```python
from build123d import *

# Parameters (mm, degrees)
FILLET1_R               = 1
FILLET2_R               = 1
BOSS_EXTRUDE1_DEPTH     = 7
CUT_EXTRUDE1_REACH      = 12.127
CUT_EXTRUDE1_END_RADIUS = 5.175
SKETCH2_R               = 1.51
SKETCH2_R_2             = 0.51
SKETCH4_R               = 0.75
CUT_EXTRUDE2_DEPTH      = 1.5


with BuildPart() as part:
    # Sketch1 → Revolve1 (revolve)
    with BuildSketch(Plane.XY, mode=Mode.PRIVATE) as revolve1_sk:
        Polygon((0, 0), (3.175, 0), (3.175, -7), (5.175, -7), (5.175, -4.640909091), (5.175, 1.5), (3.5, 1.5), (3.5, 4.5), (1.5, 4.5), (1.5, 1.5), (0, 1.5), align=None)
    revolve(revolve1_sk.sketch.rotate(Axis((0, 1.5, 0), (0, -1, 0)), 180), axis=Axis((0, 1.5, 0), (0, -1, 0)))

    # Fillet1
    fillet1_edges = [part.edges().sort_by_distance(p)[0] for p in [
        (3.5, 1.5, 0),
    ]]
    fillet(fillet1_edges, radius=FILLET1_R)

    # Fillet2
    fillet2_edges = [part.edges().sort_by_distance(p)[0] for p in [
        (5.175, 1.5, 0),
    ]]
    fillet(fillet2_edges, radius=FILLET2_R)

    # Sketch3 → Boss-Extrude1 (add)
    with BuildSketch(Plane.XZ.offset(7)):
        with BuildLine():
            Line((2.313006701, -2.175), (-2.313006701, -2.175))
            ThreePointArc((-2.313006701, -2.175), (0, -3.175), (2.313006701, -2.175))
        make_face()
    extrude(amount=-BOSS_EXTRUDE1_DEPTH)

    # Cut-Extrude1: up to this cylinder (the profile starts inside it)
    cut_extrude1_end = Plane(origin=(0, 0.120549, 0), z_dir=(0, 1, 0)) * Cylinder(CUT_EXTRUDE1_END_RADIUS, 42.18296, mode=Mode.PRIVATE)
    # Sketch2 → Cut-Extrude1 (cut, up to the surface)
    with BuildSketch(Plane.XY, mode=Mode.PRIVATE) as cut_extrude1_sk1:
        with Locations((0, -3.168930556)):
            Circle(SKETCH2_R)
    cut_extrude1_tool1 = extrude(cut_extrude1_sk1.sketch, amount=-CUT_EXTRUDE1_REACH, mode=Mode.PRIVATE) & cut_extrude1_end
    add(cut_extrude1_tool1.solids().sort_by_distance((0, -3.168931, 0))[0], mode=Mode.SUBTRACT)
    # Sketch2 → Cut-Extrude1 (cut, up to the surface)
    with BuildSketch(Plane.XY, mode=Mode.PRIVATE) as cut_extrude1_sk2:
        with Locations((0, 3.410029171)):
            Circle(SKETCH2_R_2)
    cut_extrude1_tool2 = extrude(cut_extrude1_sk2.sketch, amount=-CUT_EXTRUDE1_REACH, mode=Mode.PRIVATE) & cut_extrude1_end
    add(cut_extrude1_tool2.solids().sort_by_distance((0, 3.410029, 0))[0], mode=Mode.SUBTRACT)

    # Sketch4 → Cut-Extrude2 (cut)
    with BuildSketch(Plane.XZ):
        Circle(SKETCH4_R)
    extrude(amount=-CUT_EXTRUDE2_DEPTH, mode=Mode.SUBTRACT)


solid = part.part
```
Geometry check sheet. Reference: the model listing, model coordinates, mm. A direction names the side the tool comes from. Give positions to 0.01 mm unless a question says otherwise; leave off trailing zeros. Loops run counter-clockwise (first coordinate to the right, second up) from the corner with the lowest first, then second, coordinate; pieces in that order, holes last. Notation, with made-up numbers: M -34.75,4.5 L -10.75,4.5 A33 ccw -10.75,39.5 Z; hole C 14.25,-3.75 d11. An arc over 180 degrees is marked long. Write item = value, one per line.
(1) Sectioned sample at B-B, the plane y = -5.75. Record the cut outline in (x, z) (3 decimals).
Answer below:
outline = C 0,0 d10.35; hole M -2.313,-2.175 L 2.313,-2.175 A3.175 ccw long Z
(2) Sectioned sample at D-D, the plane y = -4.25. Record the cut outline in (x, z) (3 decimals), plus the area to 3 significant figures.
Answer below:
outline = M -2.313,-2.175 A3.175 cw long 2.313,-2.175 L 1.054,-2.175 L 1.054,-5.066 A5.175 ccw long -1.054,-5.066 L -1.054,-2.175 Z
area = 49.4 mm2
(3) Sectioned sample at A-A, the plane x = 0. State how many separate pieces and enclosed holes the cut face has, plus the area to 3 significant figures.
Answer below:
separate_pieces = 4
enclosed_holes = 0
area = 49.2 mm2
(4) Tool access check on faces 5 (the face through (-1.615, 3.514, 3.105)), 6 (the face through (0, -5, -2.175)), 7 (the face through (-1.51, -3.1, -3.65)). Record the directions out of +Z, -Z, +X, -X, +Y, -Y that give a thin tool (end or side, any length) a straight path to the whole face; none if there is none.
Answer below:
face_5 = +Y
face_6 = -Y
face_7 = -Z
(5) Sectioned sample at C-C, the plane y = -3. Record the cut outline in (x, z) (3 decimals).
Answer below:
outline = M -2.313,-2.175 A3.175 cw long 2.313,-2.175 L 1.501,-2.175 L 1.501,-4.953 A5.175 ccw long -1.501,-4.953 L -1.501,-2.175 Z
(6) Gauge pin test, flat ends, axial feed: pin 1 Ø2 at (x, z) = (0, 0) entering from +Y; pin 2 Ø2.5 at (x, z) = (-1, 0) entering from -Y; pin 3 Ø2 at (x, y) = (3.5, 1.5) entering from -Z. Record the tip position at first contact, or that the pin passes through.
Answer below:
pin_1 = 1.5
pin_2 = 0
pin_3 = -4.33
(7) Material ranges on line 1 (Y direction, x = 0, z = -3.25); line 2 (Y direction, x = -2.25, z = -2); line 3 (Y direction, x = 0.5, z = -4.5), recorded low to high. Write a range as [from, to].
Answer below:
line_1 = [-7, -4.68], [-1.66, 2.9], [3.92, 4.5]
line_2 = [0, 4.5]
line_3 = [-7, -4.59], [-1.74, 1.46]
(8) Release check for a two-part mould opening along X. For faces 1 (the face through (-0.1, -7, -2.4)), 2 (the face through (0.103, -3.549, 3.173)), 3 (the face through (1.122, -3.184, 5.052)), 4 (the face through (1, 1.5, 0)) record: released by +X, released by -X, zero draft, split by the parting line, or undercut.
Answer below:
face_1 = zero draft
face_2 = undercut
face_3 = split by the parting line
face_4 = undercut
